from build123d import *

# Parameters (mm, degrees)
SKETCH1_W          = 12.7
SKETCH1_H          = 2.413
CHAMFER1_SIZE      = 0.5953125
CUT_EXTRUDE2_DEPTH = 1.79578
SKETCH6_R          = 1.833087105
CUT_EXTRUDE3_DEPTH = 1.79578
CUT_EXTRUDE3_TAPER = 45


with BuildPart() as part:
    # Sketch1 → Revolve1 (revolve)
    with BuildSketch(Plane(origin=(0, 0, 0), x_dir=(0, 0, -1), z_dir=(1, 0, 0))):
        with Locations((8.9154, 1.2065)):
            Rectangle(SKETCH1_W, SKETCH1_H)
    revolve(axis=Axis((0, 0, -15.2654), (0, 0, 1)))

    # Chamfer1
    chamfer1_edges = [part.edges().sort_by_distance(p)[0] for p in [
        (0, -2.413, -15.2654),
    ]]
    chamfer(chamfer1_edges, length=CHAMFER1_SIZE)

    # Sketch7 → Revolve2 (revolve)
    with BuildSketch(Plane(origin=(0, 0, 0), x_dir=(0, 0, -1), z_dir=(1, 0, 0)), mode=Mode.PRIVATE) as revolve2_sk:
        with BuildLine():
            Line((2.18059, 4.5847), (2.5654, 4.5847))
            Line((2.5654, 4.5847), (2.5654, 0))
            Line((2.5654, 0), (0, 0))
            Line((0, 0), (0, 2.413))
            ThreePointArc((0, 2.413), (0.925030326, 3.664791196), (2.18059, 4.5847))
        make_face()
    revolve(revolve2_sk.sketch.rotate(Axis((0, 0, 0), (0, 0, -1)), 180), axis=Axis((0, 0, 0), (0, 0, -1)))

    # Sketch5 → Cut-Extrude2 (cut)
    with BuildSketch(Plane.XY):
        Polygon((1.5875, -0.916543552), (1.5875, 0.916543552), (0, 1.833087105), (-1.5875, 0.916543552), (-1.5875, -0.916543552), (0, -1.833087105), align=None)
    extrude(amount=-CUT_EXTRUDE2_DEPTH, mode=Mode.SUBTRACT)

    # Sketch6 → Cut-Extrude3 (cut)
    with BuildSketch(Plane.XY):
        Circle(SKETCH6_R)
    extrude(amount=-CUT_EXTRUDE3_DEPTH, taper=CUT_EXTRUDE3_TAPER, mode=Mode.SUBTRACT)


solid = part.part
Geometry check sheet. Reference: the model listing, model coordinates, mm. A direction names the side the tool comes from. Round coordinates to 2 decimals unless told otherwise and drop trailing zeros. Loops run counter-clockwise (first coordinate to the right, second up) from the corner with the lowest first, then second, coordinate; pieces in that order, holes last.
Item 1: Access from +Z, -Z, +X, -X, +Y, -Y to the whole of each face (thin tool, end or side, straight path). Record for faces 4 (the flat face through (0, 0, -15.265)), 5 (the conical face through (-0.84, 1.49, -0.12)), 6 (the flat face through (2, -2, -2.565)).
Item 2: Cross-section at D-D on y = 3.75. Record the boundary of the cut face in (x, z), then the cut area to 3 significant figures.
Item 3: Cross-section at C-C on x = 3.25. Record the boundary of the cut face in (y, z), then the cut area to 3 significant figures.
Item 4: Gauge pin test, flat ends, axial feed: pin 1 (1.5 mm diameter, centred on y = 2.5, z = -8, fed in from -X); pin 2 (2 mm diameter, centred on y = 0, z = -4.5, fed in from -X); pin 3 (1.5 mm diameter, centred on x = 2, z = -9, fed in from -Y). Record the tip position at first contact, or that the pin passes through.
Item 5: Cross-section at A-A on y = 0. Record the boundary of the cut face in (x, z).
Item 6: Cross-section at B-B on z = -4. Record the boundary of the cut face in (x, y), then the cut area to 3 significant figures.
Item 7: Thickness scan on line 1 (Z direction, x = 0.5, y = 1.25); line 2 (X direction, y = 0.25, z = -10.75); line 3 (Z direction, x = -1.75, y = 2). Record the ranges inside material, lowest first.
Item 8: Mould release check, pull along X, two halves, no side actions. Record for faces 1 (the flat face through (-2, 0, 0)), 2 (the cylindrical face through (4.476, 0.994, -2.376)), 3 (the flat face through (-0.8, -1.37, -0.89)): pulls with the +X half, pulls with the -X half, needs draft (parallel to the pull), parting line crosses it, or undercut.
Answer sheet:
1. face 4: -Z, +X, -X, +Y, -Y
1. face 5: +Z
1. face 6: -Z
2. outline: (-2.64, -2.57) - (2.64, -2.57) - (2.64, -2.18) arc R3.56 ccw to (-2.64, -2.18) - close
2. area: 6.29 mm2
3. outline: (-3.23, -2.57) - (3.23, -2.57) - (3.23, -2.18) arc R4.02 ccw to (-3.23, -2.18) - close
3. area: 9.86 mm2
4. pin 1: stops at x = -1.66
4. pin 2: stops at x = -2.41
4. pin 3: stops at y = -2.06
5. outline: (-4.58, -2.57) - (-2.41, -2.57) - (-2.41, -14.67) - (-1.82, -15.27) - (1.82, -15.27) - (2.41, -14.67) - (2.41, -2.57) - (4.58, -2.57) - (4.58, -2.18) arc R5.17 ccw to (2.41, 0) - (1.83, 0) - (1.59, -0.25) - (1.59, -1.8) - (-1.59, -1.8) - (-1.59, -0.25) - (-1.83, 0) - (-2.41, 0) arc R5.17 ccw to (-4.58, -2.18) - close
6. outline: circle Ø4.83 at (0, 0)
6. area: 18.3 mm2
7. line 1: z = -15.27 to -1.8
7. line 2: x = -2.4 to 2.4
7. line 3: z = -2.57 to -0.14
8. face 1: needs draft
8. face 2: parting line crosses it
8. face 3: undercut
